Part model, mm, in its own coordinate system. A direction names the side the tool comes from. Give positions to 0.01 mm unless a question says otherwise; leave off trailing zeros. Order: outer loops, then holes, each group sorted by start corner. A loop starts at its lowest first (then second) coordinate and runs counter-clockwise, first axis right, second up. Notation, with made-up numbers: (64.25, 45) - (86.25, 45) arc R10 ccw to (86.25, 57) - close; hole circle Ø4 at (88.5, 8.25). An arc over 180 degrees is marked (long way). Use a Markdown table: item, result. Add a question column.
from build123d import *

# Parameters (mm, degrees)
SKETCH2_W               = 55
SKETCH2_H               = 38
BOSS_EXTRUDE1_DEPTH     = 2
SKETCH3_R               = 3.2
BOSS_EXTRUDE2_DEPTH     = 10
SKETCH4_R               = 3.6
BOSS_EXTRUDE3_DEPTH     = 1
CHAMFER1_SIZE           = 3
SKETCH5_W               = 2
SKETCH5_H               = 10.684354826
CUT_EXTRUDE1_DEPTH      = 6
CHAMFER2_SIZE           = 10
CUT_EXTRUDE2_DEPTH      = 35.889110049
CUT_EXTRUDE2_DEPTH_BACK = 35.889110049
SKETCH8_W               = 9.45
SKETCH8_H               = 2
FILLET2_R               = 16


with BuildPart() as part:
    # Sketch2 → Boss-Extrude1 (new body)
    with BuildSketch(Plane(origin=(0, 0, 0), x_dir=(1, 0, 0), z_dir=(0, 1, 0))):
        Rectangle(SKETCH2_W, SKETCH2_H)
    extrude(amount=BOSS_EXTRUDE1_DEPTH)

    # Sketch3 → Boss-Extrude2 (add)
    with BuildSketch(Plane(origin=(0, 0, 0), x_dir=(1, 0, 0), z_dir=(0, 1, 0))):
        with Locations(Location((-16.675, 3.65, 0), (0, 0, 270))):
            Circle(SKETCH3_R)
        with Locations(Location((16.675, 3.65, 0), (0, 0, 90))):
            Circle(SKETCH3_R)
    extrude(amount=BOSS_EXTRUDE2_DEPTH)

    # Sketch4 → Boss-Extrude3 (add)
    with BuildSketch(Plane(origin=(0, 10, 0), x_dir=(1, 0, 0), z_dir=(0, 1, 0))):
        with Locations(Location((-16.675, 3.65, 0), (0, 0, 270))):
            Circle(SKETCH4_R)
        with Locations(Location((16.675, 3.65, 0), (0, 0, 90))):
            Circle(SKETCH4_R)
    extrude(amount=-BOSS_EXTRUDE3_DEPTH)

    # Chamfer1
    # the kernel refuses this chamfer: 3 mm, written as the material it adds along each edge
    with BuildSketch(Plane(origin=(16.675, 9, -3.65), x_dir=(0, 0, -1), z_dir=(-1, 0, 0))) as chamfer1_piece_1_section:
        Polygon((3.2, CHAMFER1_SIZE), (3.2 + CHAMFER1_SIZE, 0), (3.2, 0), align=None)
    chamfer1_piece_1 = revolve(axis=Axis((16.675, 9, -3.65), (0, -1, 0)), mode=Mode.PRIVATE)
    chamfer1_piece_1 = chamfer1_piece_1 & Plane(origin=(16.675, 6.179265151, -3.65), x_dir=(0, 0, -1), z_dir=(0, 1, 0)) * Cylinder(3.6, 25, mode=Mode.PRIVATE)
    add(chamfer1_piece_1)
    with BuildSketch(Plane(origin=(-16.675, 9, -3.65), x_dir=(0, 0, 1), z_dir=(1, 0, 0))) as chamfer1_piece_2_section:
        Polygon((3.2, CHAMFER1_SIZE), (3.2 + CHAMFER1_SIZE, 0), (3.2, 0), align=None)
    chamfer1_piece_2 = revolve(axis=Axis((-16.675, 9, -3.65), (0, -1, 0)), mode=Mode.PRIVATE)
    chamfer1_piece_2 = chamfer1_piece_2 & Plane(origin=(-16.675, 6.179265151, -3.65), x_dir=(0, 0, 1), z_dir=(0, 1, 0)) * Cylinder(3.6, 25, mode=Mode.PRIVATE)
    add(chamfer1_piece_2)

    # Sketch5 → Cut-Extrude1 (cut)
    with BuildSketch(Plane(origin=(0, 10, 0), x_dir=(1, 0, 0), z_dir=(0, 1, 0))):
        with Locations((16.675, 3.65)):
            Rectangle(SKETCH5_W, SKETCH5_H)
        with Locations((-16.675, 3.65)):
            Rectangle(SKETCH5_W, SKETCH5_H)
    extrude(amount=-CUT_EXTRUDE1_DEPTH, mode=Mode.SUBTRACT)

    # Chamfer2
    chamfer2_edges = [part.edges().sort_by_distance(p)[0] for p in [
        (-27.5, 1, -19),
        (27.5, 1, -19),
    ]]
    chamfer(chamfer2_edges, length=CHAMFER2_SIZE)

    # Sketch8 → Cut-Extrude2 (cut, two sides: drawn at the far end of the back side and taken through both)
    with BuildSketch(Plane.ZY.offset(-CUT_EXTRUDE2_DEPTH_BACK)):
        with Locations((14.275, 1)):
            Rectangle(SKETCH8_W, SKETCH8_H)
    extrude(amount=CUT_EXTRUDE2_DEPTH + CUT_EXTRUDE2_DEPTH_BACK, mode=Mode.SUBTRACT)

    # Fillet2
    fillet2_edges = [part.edges().sort_by_distance(p)[0] for p in [
        (27.5, 1, 9.55),
        (-27.5, 1, 9.55),
    ]]
    fillet(fillet2_edges, radius=FILLET2_R)


solid = part.part
1. Tool access for faces 4 (the face through (-17.675, 7, -4)), 5 (the face through (19.51, 3.97, -5.13)), 6 (the face through (13.076, 8.225, -3.715)), 7 (the face through (-20.274, 8.225, -3.715)): list every direction of +Z, -Z, +X, -X, +Y, -Y with a clear straight run to the whole face (end or side of a thin tool).
2. Mould opens along X. For faces 1 (the face through (-19.988, 6.114, -3.59)), 2 (the face through (-19.51, 3.97, -2.17)), 3 (the face through (0, 1, -19)) say: released by +X, released by -X, zero draft, split by the parting line, or undercut.
3. Pin check, flat tips, straight feed: P1, Ø0.6, axis at x = -16.5, z = -3, coming from the +Y side; P2, Ø3, axis at y = 6.5, z = -4.5, coming from the +X side (3 decimals); P3, Ø8, axis at x = 1, z = 2, coming from the +Y side. Stop position of each tip, or through.
4. Drill centre lines: probe 1 along Y at (x, z) = (-14, -0.25); probe 2 along X at (y, z) = (6.75, -0.75) (3 decimals); probe 3 along X at (y, z) = (7, -5) (3 decimals). Where is each one in solid material? Low to high. Write a range as [from, to].
5. Cut at D-D (x = -2.5). Write the cut outline in (y, z).
6. Cut at B-B (y = 1). Write the cut outline in (x, z), plus the area to 3 significant figures.
7. Cut at C-C (z = -15.5). Write the cut outline in (x, y), plus the area to 3 significant figures.
8. Cut at A-A (y = 8). Write the cut outline in (x, z) (3 decimals).
Responses:
| question | item | result |
|---|---|---|
| 1 | face 4 | +Z, -Z, +Y |
| 1 | face 5 | none |
| 1 | face 6 | +Y |
| 1 | face 7 | -X, +Y |
| 2 | face 1 | released by -X |
| 2 | face 2 | undercut |
| 2 | face 3 | zero draft |
| 3 | P1 | stops at y = 4 |
| 3 | P2 | stops at x = 20.275 |
| 3 | P3 | stops at y = 2 |
| 4 | probe 1 | y = [0, 2] |
| 4 | probe 2 | x = [-18.808, -17.675], [-15.675, -14.542], [14.542, 15.675], [17.675, 18.808] |
| 4 | probe 3 | x = [-20.012, -17.675], [-15.675, -13.338], [13.338, 15.675], [17.675, 20.012] |
| 5 | outline | (0, -19) - (2, -19) - (2, 9.55) - (0, 9.55) - close |
| 6 | outline | (-27.5, -9) - (-17.5, -19) - (17.5, -19) - (27.5, -9) - (27.5, -6.45) arc R16 ccw to (11.5, 9.55) - (-11.5, 9.55) arc R16 ccw to (-27.5, -6.45) - close |
| 6 | area | 1,360 mm² |
| 7 | outline | (-21, 0) - (21, 0) - (21, 2) - (-21, 2) - close |
| 7 | area | 84.0 mm² |
| 8 | outline | (-17.675, -7.108) - (-17.675, -0.192) arc R3.6 ccw to start; (-15.675, -7.108) arc R3.6 ccw to (-15.675, -0.192) - close; (15.675, -7.108) - (15.675, -0.192) arc R3.6 ccw to start; (17.675, -7.108) arc R3.6 ccw to (17.675, -0.192) - close |
